```python
from build123d import *

# Parameters (mm, degrees)
SKETCH_R           = 70
SKETCH_R_2         = 57.5
PAD_DEPTH          = 40
SKETCH001_W        = 40
SKETCH001_H        = 30
PAD001_DEPTH       = 40
PAD001_FACE1_W     = 31.626028
PAD001_FACE1_H     = 40
POCKET_DEPTH       = 10
POCKET_FACE3_W     = 31.626028
POCKET_FACE3_H     = 40
POCKET001_DEPTH    = 10
POCKET001_FACE6_W  = 31.626028
POCKET001_FACE6_H  = 40
POCKET002_DEPTH    = 9
POCKET002_FACE11_W = 31.626028
POCKET002_FACE11_H = 40
POCKET003_DEPTH    = 9
SKETCH002_R        = 70
PAD002_DEPTH       = 40
SKETCH003_R        = 57.5
POCKET004_DEPTH    = 522
SKETCH004_W        = 150
SKETCH004_H        = 100
POCKET005_DEPTH    = 40
FILLET_R           = 8
FILLET001_R        = 3
SKETCH005_R        = 2.75
POCKET006_DEPTH    = 20


with BuildPart() as part:
    # Sketch → Pad (new body)
    with BuildSketch(Plane.XY):
        Circle(SKETCH_R)
        Circle(SKETCH_R_2, mode=Mode.SUBTRACT)
    extrude(amount=PAD_DEPTH)

    # Sketch001 (on Face4 of Pad) → Pad001 (join)
    with BuildSketch(Plane.XY.offset(40)):
        with Locations((-80, 0)):
            Rectangle(SKETCH001_W, SKETCH001_H)
        with Locations((80, 0)):
            Rectangle(SKETCH001_W, SKETCH001_H)
    extrude(amount=-PAD001_DEPTH)

    # Pad001 Face1 → Pocket (cut)
    with BuildSketch(Plane(origin=(84.186986, 15, 20), x_dir=(1, 0, 0), z_dir=(0, 1, 0))):
        Rectangle(PAD001_FACE1_W, PAD001_FACE1_H)
    extrude(amount=-POCKET_DEPTH, mode=Mode.SUBTRACT)

    # Pocket Face3 → Pocket001 (cut)
    with BuildSketch(Plane(origin=(-84.186986, 15, 20), x_dir=(1, 0, 0), z_dir=(0, 1, 0))):
        Rectangle(POCKET_FACE3_W, POCKET_FACE3_H)
    extrude(amount=-POCKET001_DEPTH, mode=Mode.SUBTRACT)

    # Pocket001 Face6 → Pocket002 (cut)
    with BuildSketch(Plane(origin=(-84.186986, 5, 20), x_dir=(1, 0, 0), z_dir=(0, 1, 0))):
        Rectangle(POCKET001_FACE6_W, POCKET001_FACE6_H)
    extrude(amount=-POCKET002_DEPTH, mode=Mode.SUBTRACT)

    # Pocket002 Face11 → Pocket003 (cut)
    with BuildSketch(Plane(origin=(84.186986, 5, 20), x_dir=(1, 0, 0), z_dir=(0, 1, 0))):
        Rectangle(POCKET002_FACE11_W, POCKET002_FACE11_H)
    extrude(amount=-POCKET003_DEPTH, mode=Mode.SUBTRACT)

    # Sketch002 (on Face2 of Pocket003) → Pad002 (join)
    with BuildSketch(Plane(origin=(0, 0, 0), x_dir=(1, 0, 0), z_dir=(0, 0, -1))):
        Circle(SKETCH002_R)
    extrude(amount=-PAD002_DEPTH)

    # Sketch003 (on Face8 of Pad002) → Pocket004 (cut)
    with BuildSketch(Plane(origin=(0, 0, 0), x_dir=(1, 0, 0), z_dir=(0, 0, -1))):
        Circle(SKETCH003_R)
    extrude(amount=-POCKET004_DEPTH, mode=Mode.SUBTRACT)

    # Sketch004 (on Face5 of Pocket004) → Pocket005 (cut)
    with BuildSketch(Plane(origin=(0, 0, 0), x_dir=(1, 0, 0), z_dir=(0, 0, -1))):
        with Locations((0, -46)):
            Rectangle(SKETCH004_W, SKETCH004_H)
    extrude(amount=-POCKET005_DEPTH, mode=Mode.SUBTRACT)

    # Fillet
    fillet_edges = [part.edges().sort_by_distance(p)[0] for p in [
        (-68.373972, -15, 20),
        (68.373972, -15, 20),
    ]]
    fillet(fillet_edges, radius=FILLET_R)

    # Fillet001
    fillet001_edges = [part.edges().sort_by_distance(p)[0] for p in [
        (100, -15, 20),
        (100, -4, 20),
        (-100, -15, 20),
        (-100, -4, 20),
    ]]
    fillet(fillet001_edges, radius=FILLET001_R)

    # Sketch005 (on Face10 of Fillet001) → Pocket006 (cut)
    with BuildSketch(Plane.XZ.offset(15)):
        with Locations((-88, 30)):
            Circle(SKETCH005_R)
        with Locations((-88, 10)):
            Circle(SKETCH005_R)
        with Locations((88, 30)):
            Circle(SKETCH005_R)
        with Locations((88, 10)):
            Circle(SKETCH005_R)
    extrude(amount=-POCKET006_DEPTH, mode=Mode.SUBTRACT)


solid = part.part
```
Check sheet for the modelled part. Datum: model origin and axes. Units: mm. A direction names the side the tool comes from. Give positions to 0.01 mm unless a question says otherwise; leave off trailing zeros. Order: outer loops, then holes, each group sorted by start corner. A loop starts at its lowest first (then second) coordinate and runs counter-clockwise, first axis right, second up. Notation, with made-up numbers: (84, 58.25) -> (140, 58.25) arc R25 ccw to (140, 80.25) -> close; hole circle Ø4 at (19, -22.5). An arc over 180 degrees is marked (long way). Use CSV: the item, a comma, the result in double quotes. Start each with the question number.
1) Sectioned sample at C-C, the plane x = 88. Record the boundary of the cut face in (y, z).
2) Sectioned sample at A-A, the plane z = 10. Record the boundary of the cut face in (x, y), plus the area to 3 significant figures.
3) Set-up check for faces 5 (the face through (-86, -15, 20)), 6 (the face through (85.253, -9.577, 30.121)), 7 (the face through (86, -15, 20)): record each of +Z, -Z, +X, -X, +Y, -Y from which the full face is reachable in a straight line by a thin tool's end or side.
4) Sectioned sample at D-D, the plane y = -47. Record the boundary of the cut face in (x, z).
5) Mould release check, pull along Z, two halves, no side actions. Record for faces 1 (the face through (85.253, -9.577, 10.121)), 2 (the face through (-90.747, -9.577, 30.121)), 3 (the face through (7, -59, 0)), 4 (the face through (1.208, -57.487, 19.72)): released by +Z, released by -Z, zero draft, split by the parting line, or undercut.
6) Go/stop test with flat-tipped pins: P1, Ø3.5, axis at x = -88, z = 10, coming from the +Y side; P2, Ø12, axis at y = -43, z = 21.5, coming from the -X side; P3, Ø1, axis at y = -14.5, z = 33, coming from the +X side. Record where each tip stops, or that it passes through.
7) Material ranges on line 1 (Z direction, x = -88, y = -5); line 2 (Y direction, x = -2, z = 2); line 3 (X direction, y = -24.5, z = 33), recorded low to high. Write a range as from..to.
8) Sectioned sample at B-B, the plane y = -9.5. Record the boundary of the cut face in (x, z), plus the area to 3 significant figures.
Recorded:
1,outline,"(-15, 0) -> (-4, 0) -> (-4, 7.25) -> (-15, 7.25) -> close; (-15, 12.75) -> (-4, 12.75) -> (-4, 27.25) -> (-15, 27.25) -> close; (-15, 32.75) -> (-4, 32.75) -> (-4, 40) -> (-15, 40) -> close"
2,outline,"(-100, -12) arc R3 ccw to (-97, -15) -> (-90.75, -15) -> (-90.75, -4) -> (-97, -4) arc R3 ccw to (-100, -7) -> close; (-85.25, -15) -> (-74.53, -15) arc R8 cw to (-66.89, -20.64) arc R70 ccw to (66.89, -20.64) arc R8 cw to (74.53, -15) -> (85.25, -15) -> (85.25, -4) -> (57.36, -4) arc R57.5 cw to (-57.36, -4) -> (-85.25, -4) -> close; (90.75, -15) -> (97, -15) arc R3 ccw to (100, -12) -> (100, -7) arc R3 ccw to (97, -4) -> (90.75, -4) -> close"
2,area,"2,960 mm2"
3,face 5,"+Z, -Z, -X, -Y"
3,face 6,"+Y, -Y"
3,face 7,"+Z, -Z, +X, -Y"
4,outline,"(-51.87, 0) -> (-33.12, 0) -> (-33.12, 40) -> (-51.87, 40) -> close; (33.12, 0) -> (51.87, 0) -> (51.87, 40) -> (33.12, 40) -> close"
5,face 1,"undercut"
5,face 2,"undercut"
5,face 3,"released by -Z"
5,face 4,"zero draft"
6,P1,"through"
6,P2,"x = -59.42"
6,P3,"x = 99.24"
7,line 1,"0..7.25, 12.75..27.25, 32.75..40"
7,line 2,"-69.97..-57.47"
7,line 3,"-65.57..-52.02, 52.02..65.57"
8,outline,"(-100, 0) -> (-56.71, 0) -> (-56.71, 40) -> (-100, 40) -> close; (56.71, 0) -> (100, 0) -> (100, 40) -> (56.71, 40) -> close; hole circle Ø5.5 at (-88, 10); hole circle Ø5.5 at (-88, 30); hole circle Ø5.5 at (88, 10); hole circle Ø5.5 at (88, 30)"
8,area,"3,370 mm2"
